from build123d import *

# Parameters (mm, degrees)
F1_DEPTH = 63.5
F0_W     = 27.0158293307
F0_H     = 19.05
F2_DEPTH = 25.4
F3_DEPTH = 7.9375
F5_R     = 5.08


with BuildPart() as f1:
    # F0 (on Front) → F1 (new body, symmetric)
    with BuildSketch(Plane.XZ):
        Polygon((41.275, -9.525), (41.275, 9.525), (22.225, 9.525), (-41.275, 9.525), (-41.275, -9.525), align=None)
    extrude(amount=F1_DEPTH, both=True)

    # F0 (on Front) → F2 (join, symmetric)
    with BuildSketch(Plane.XZ):
        with BuildLine():
            Line((22.225, 9.525), (41.275, 9.525))
            Line((41.275, 9.525), (41.275, 40.7823575326))
            ThreePointArc((41.275, 40.7823575326), (45.4239723265, 51.4835677445), (55.7022, 56.5912))
            Line((55.7022, 56.5912), (58.7091706693, 56.5912))
            Line((58.7091706693, 56.5912), (58.7091706693, 75.6412))
            Line((58.7091706693, 75.6412), (55.0013430169, 75.6412))
            ThreePointArc((55.0013430169, 75.6412), (31.7059685768, 64.7063390142), (22.225, 40.7823575326))
            Line((22.225, 40.7823575326), (22.225, 9.525))
        make_face()
        with Locations((72.2170853347, 66.1162)):
            Rectangle(F0_W, F0_H)
    extrude(amount=F2_DEPTH, both=True)

    # F0 (on Front) → F3 (join, symmetric)
    with BuildSketch(Plane.XZ):
        with BuildLine():
            Line((-41.275, 9.525), (22.225, 9.525))
            Line((22.225, 9.525), (22.225, 40.7823575326))
            ThreePointArc((22.225, 40.7823575326), (31.7059685768, 64.7063390142), (55.0013430169, 75.6412))
            Line((55.0013430169, 75.6412), (58.7091706693, 75.6412))
            Line((58.7091706693, 75.6412), (58.7091706693, 80.5059267402))
            add(Edge.make_bspline(
                [(-41.275, 9.525), (-31.0757625848, 34.9992662668), (-12.4977082014, 76.490201056), (58.7091706693, 80.5059267402)],
                knots=[0, 0, 0, 0, 122.6178059881, 122.6178059881, 122.6178059881, 122.6178059881], degree=3))
        make_face()
    extrude(amount=F3_DEPTH, both=True)

    # F0 (on Front) → F4 (revolve)
    with BuildSketch(Plane.XZ):
        Polygon((109.5091706693, 80.5059267402), (85.725, 80.5059267402), (85.725, 75.6412), (85.725, 56.5912), (85.725, 51.9309267402), (109.5091706693, 51.9309267402), align=None)
    revolve(axis=Axis((85.725, 0, 66.2184267402), (0, 0, -1)))

    # F5
    f5_edges = [f1.edges().sort_by_distance(p)[0] for p in [
        (41.275, 63.5, 0),
        (-41.275, 63.5, 0),
        (-41.275, -63.5, 0),
        (41.275, -63.5, 0),
    ]]
    fillet(f5_edges, radius=F5_R)


solid = f1.part
Geometry check sheet. Reference: the model listing, model coordinates, mm. A direction names the side the tool comes from. Give positions to 0.01 mm unless a question says otherwise; leave off trailing zeros. Order: outer loops, then holes, each group sorted by start corner. A loop starts at its lowest first (then second) coordinate and runs counter-clockwise, first axis right, second up. Notation, with made-up numbers: M -32,84.5 L 5,84.5 A10 cw 5,92.5 Z; hole C -12.75,74 d1. An arc over 180 degrees is marked long. Use a Markdown table: item, result.
Item 1: Depth check by flat-ended pin: P1, Ø1.5, axis at y = -21.5, z = 63, coming from the +X side; P2, Ø25, axis at y = 22.5, z = 13.5, coming from the +X side (3 decimals); P3, Ø19, axis at y = 17.5, z = 29.5, coming from the -X side (3 decimals). Enter the tip coordinate at first touch or a pass-through.
Answers follow:
| item | result |
|---|---|
| P1 | stops at x = 97.35 |
| P2 | stops at x = 41.275 |
| P3 | stops at x = 22.225 |
Item 2: Section check A-A (y = 20). Record the cut outline in (x, z) (3 decimals), and give its area (3 significant figures).
Answers follow:
| item | result |
|---|---|
| outline | M -41.275,-9.525 L 41.275,-9.525 L 41.275,40.782 A15.875 cw 55.702,56.591 L 72.853,56.591 L 72.853,51.931 L 98.597,51.931 L 98.597,80.506 L 72.853,80.506 L 72.853,75.641 L 55.001,75.641 A34.925 ccw 22.225,40.782 L 22.225,9.525 L -41.275,9.525 Z |
| area | 3,960 mm2 |
Item 3: Section check B-B (y = 37.5). Record the cut outline in (x, z) (3 decimals), and give its area (3 significant figures).
Answers follow:
| item | result |
|---|---|
| outline | M -41.275,-9.525 L 41.275,-9.525 L 41.275,9.525 L -41.275,9.525 Z |
| area | 1,570 mm2 |
Item 4: Tool access check on faces 1 (the flat face through (22.225, -17, 25)), 2 (the flat face through (41.275, -1, 10)), 3 (the flat face through (39, 25.4, 50)), 4 (the flat face through (8, 7.938, 38)). Record the directions out of +Z, -Z, +X, -X, +Y, -Y that give a thin tool (end or side, any length) a straight path to the whole face; none if there is none.
Answers follow:
| item | result |
|---|---|
| face 1 | +Z, -X, -Y |
| face 2 | -Z, +X, +Y, -Y |
| face 3 | +Z, +X, -X, +Y |
| face 4 | +Z, -X, +Y |
Item 5: Material ranges on line 1 along X through (y, z) = (-9, 29) (3 decimals); line 2 along Z through (x, y) = (8, -10) (3 decimals); line 3 along Y through (x, z) = (81, 68.5), recorded low to high.
Answers follow:
| item | result |
|---|---|
| line 1 | x = 22.225 to 41.275 |
| line 2 | z = -9.525 to 9.525 |
| line 3 | y = -25.4 to 25.4 |
Item 6: Draft check along X on faces 5 (the flat face through (-1, 63.5, 0)), 6 (the flat face through (58.709, 0, 78)), 7 (the cylindrical face through (31.96, -16.791, 64.974)). Enter one of: +X half, -X half, draft (parallel to the pull), parting line (faces both ways), or undercut.
Answers follow:
| item | result |
|---|---|
| face 5 | draft |
| face 6 | undercut |
| face 7 | -X half |
